Geometry: see drawing. Coordinates: mm, zero at the bounding-box minimum. Round coordinates to 2 decimals unless told otherwise and drop trailing zeros. Write each loop counter-clockwise with the first axis right and the second up, starting at its lowest first coordinate (ties: lowest second). Pieces come first, ordered by that corner, then holes. Notation, with made-up numbers: M 43,25.25 L 62,25.25 A36 cw 62,62.25 Z; hole C -15.5,-14 d2. An arc over 180 degrees is marked long. Write each question's results on one line, items separated by ' | '. Start each with the question number.
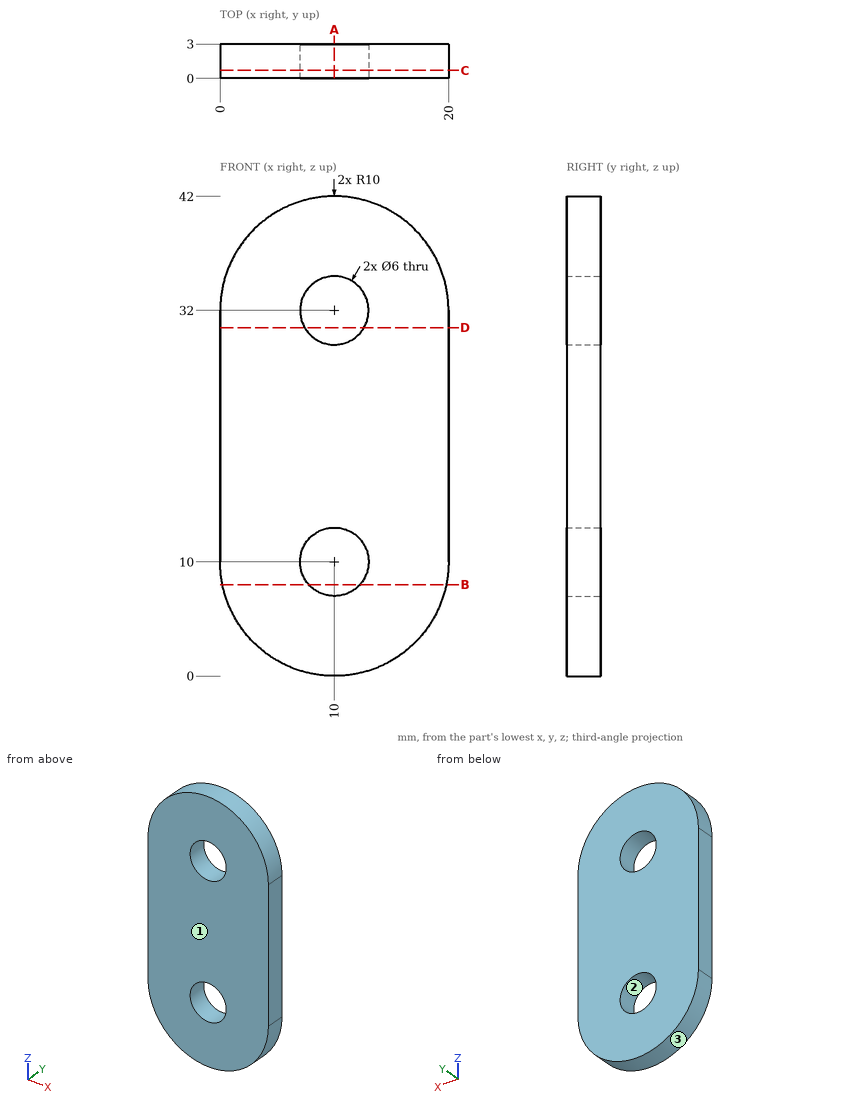
1. Draft query along Z for the marked faces 1, 2 and 3. Return one class per face: +Z half, -Z half, draft (parallel to the pull), parting line (faces both ways), or undercut.
2. Cut plane D-D on z = 30.5. Output: boundary loops of the cut face in (x, y).
3. Contact query for flat-ended pins moving along their axis: P1, Ø3.5, axis at x = 10, z = 10, coming from the +Y side; P2, Ø1.5, axis at x = 6.5, y = 1, coming from the +Z side. Output: stop coordinate, or through.
4. Cut plane B-B on z = 8. Output: boundary loops of the cut face in (x, y).
5. Cut plane A-A on x = 10. Output: boundary loops of the cut face in (y, z).
6. Cut plane C-C on y = 0.7. Output: boundary loops of the cut face in (x, z).
7. Line query: L1, parallel to Z at x = 10, y = 0.65; L2, parallel to Z at x = 7.5, y = 1.05; L3, parallel to X at y = 1.55, z = 10. Output: solid intervals per line, ascending. Write a range as from..to.
Answers follow:
1) face 1: draft | face 2: undercut | face 3: -Z half
2) outline: M 0,0 L 7.4,0 L 7.4,3 L 0,3 Z; M 12.6,0 L 20,0 L 20,3 L 12.6,3 Z
3) P1: passes through | P2: stops at z = 41.61
4) outline: M 0.2,0 L 7.76,0 L 7.76,3 L 0.2,3 Z; M 12.24,0 L 19.8,0 L 19.8,3 L 12.24,3 Z
5) outline: M 0,0 L 3,0 L 3,7 L 0,7 Z; M 0,13 L 3,13 L 3,29 L 0,29 Z; M 0,35 L 3,35 L 3,42 L 0,42 Z
6) outline: M 0,10 A10 ccw 20,10 L 20,32 A10 ccw 0,32 Z; hole C 10,10 d6; hole C 10,32 d6
7) L1: z = 0..7, 13..29, 35..42 | L2: z = 0.32..8.34, 11.66..30.34, 33.66..41.68 | L3: x = 0..7, 13..20
